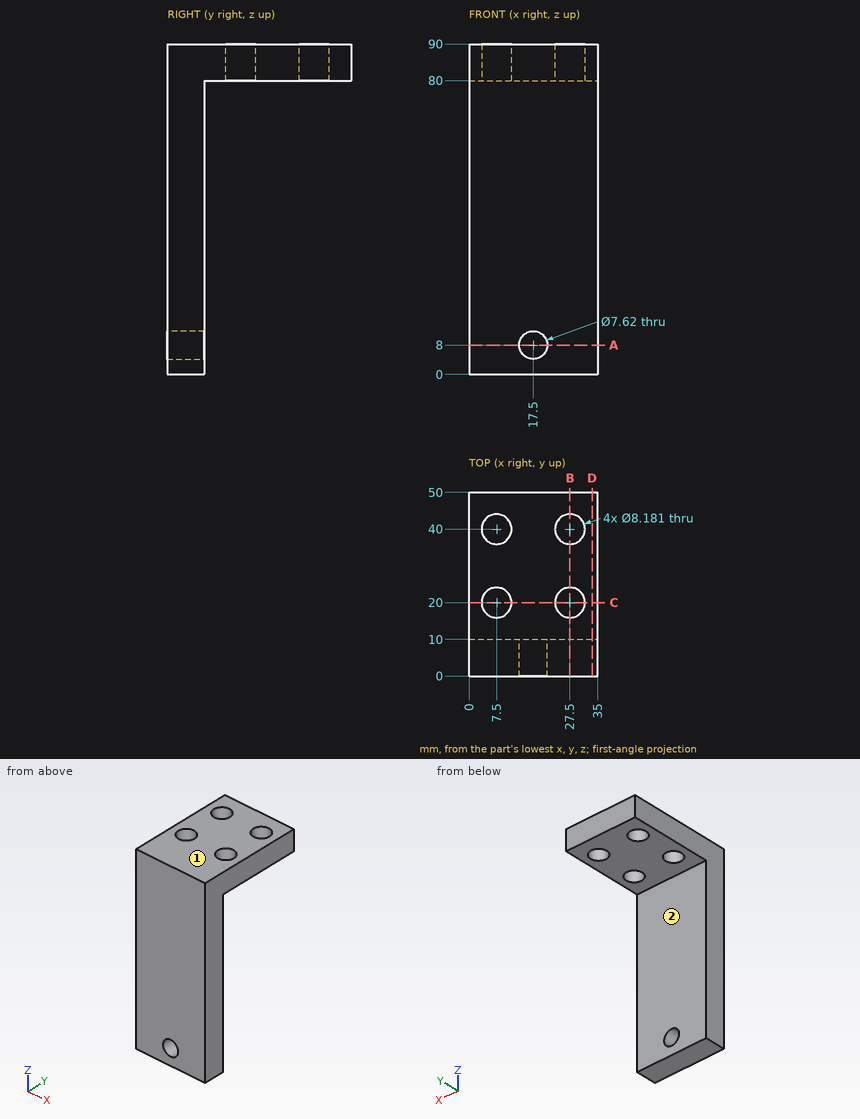
Source: three-view drawing plus pictorial views. Frame: mm from the lowest corner of the part. A direction names the side the tool comes from. Round coordinates to 2 decimals unless told otherwise and drop trailing zeros. Loops run counter-clockwise (first coordinate to the right, second up) from the corner with the lowest first, then second, coordinate; pieces in that order, holes last.
Q1. Section A-A on z = 8. Return loops of the section in (x, y).
Q2. Section D-D on x = 33.5. Return loops of the section in (y, z).
Q3. Material intervals for L1, parallel to X at y = 20, z = 83.25; L2, parallel to Y at x = 27.5, z = 86; L3, parallel to Z at x = 18, y = 47, sorted ascending.
Q4. Section C-C on y = 20. Return loops of the section in (x, z).
Q5. Pin query (flat end, axial travel): P1, Ø17.5, axis at x = 22.5, z = 54, coming from the +Y side; P2, Ø10.5, axis at x = 16.5, y = 26, coming from the -Z side; P3, Ø6.5, axis at x = 27.5, y = 40, coming from the -Z side. Return the tip coordinate at first contact, or that it passes through.
Q6. Access query for the marked faces 1 and 2. Directions: +Z, -Z, +X, -X, +Y, -Y. A direction counts if a zero-diameter tool reaches every point of the face in a straight line with its end or side. Return the directions, or none.
Q7. Section B-B on x = 27.5. Return loops of the section in (y, z).
Evaluation:
1. outline: (0, 0) - (13.69, 0) - (13.69, 10) - (0, 10) - close; (21.31, 0) - (35, 0) - (35, 10) - (21.31, 10) - close
2. outline: (0, 0) - (10, 0) - (10, 80) - (50, 80) - (50, 90) - (0, 90) - close
3. L1: x = 0 to 3.41, 11.59 to 23.41, 31.59 to 35
3. L2: y = 0 to 15.91, 24.09 to 35.91, 44.09 to 50
3. L3: z = 80 to 90
4. outline: (0, 80) - (3.41, 80) - (3.41, 90) - (0, 90) - close; (11.59, 80) - (23.41, 80) - (23.41, 90) - (11.59, 90) - close; (31.59, 80) - (35, 80) - (35, 90) - (31.59, 90) - close
5. P1: stops at y = 10
5. P2: stops at z = 80
5. P3: passes through
6. face 1: +Z, +X, -X, +Y, -Y
6. face 2: -Z, +X, -X, +Y
7. outline: (0, 0) - (10, 0) - (10, 80) - (15.91, 80) - (15.91, 90) - (0, 90) - close; (24.09, 80) - (35.91, 80) - (35.91, 90) - (24.09, 90) - close; (44.09, 80) - (50, 80) - (50, 90) - (44.09, 90) - close
